Build history of the part. All positions in model axes, mm. A direction names the side the tool comes from. Coordinates: 2 decimals unless noted, no trailing zeros. Order: outer loops, then holes, each group sorted by start corner. A loop starts at its lowest first (then second) coordinate and runs counter-clockwise, first axis right, second up. Notation, with made-up numbers: (29.25, 56.25) - (48.25, 56.25) arc R13 cw to (48.25, 69.25) - close; hole circle Ø8 at (37, -10.5). An arc over 180 degrees is marked (long way). One line per item, written item: value.
from build123d import *

# Parameters (mm, degrees)
SKETCH1_W           = 120
SKETCH1_H           = 120
BOSS_EXTRUDE1_DEPTH = 50
SKETCH3_R           = 35
BOSS_EXTRUDE2_DEPTH = 25
SKETCH4_R           = 25
CUT_EXTRUDE1_DEPTH  = 76
FILLET1_R           = 10
SHELL1_T            = -2
FILLET8_R           = 1.5
FILLET9_R           = 5


with BuildPart() as part:
    # Sketch1 → Boss-Extrude1 (new body)
    with BuildSketch(Plane.XY):
        with Locations((60, 60)):
            Rectangle(SKETCH1_W, SKETCH1_H)
    extrude(amount=BOSS_EXTRUDE1_DEPTH)

    # Sketch3 → Boss-Extrude2 (add)
    with BuildSketch(Plane.XY.offset(50)):
        with Locations((60, 60)):
            Circle(SKETCH3_R)
    extrude(amount=BOSS_EXTRUDE2_DEPTH)

    # Sketch4 → Cut-Extrude1 (cut, through all)
    with BuildSketch(Plane.XY.offset(75)):
        with Locations((60, 60)):
            Circle(SKETCH4_R)
    extrude(amount=-CUT_EXTRUDE1_DEPTH, mode=Mode.SUBTRACT)

    # Fillet1
    fillet1_edges = [part.edges().sort_by_distance(p)[0] for p in [
        (0, 120, 25),
        (120, 120, 25),
        (120, 0, 25),
        (0, 0, 25),
    ]]
    fillet(fillet1_edges, radius=FILLET1_R)

    # Shell1
    shell1_openings = [part.faces().sort_by_distance(p)[0] for p in [
        (85, 60, 0),
    ]]
    offset(amount=SHELL1_T, openings=shell1_openings, kind=Kind.INTERSECTION)

    # Fillet8
    fillet8_edges = [part.edges().sort_by_distance(p)[0] for p in [
        (25, 60, 75),
        (35, 60, 75),
    ]]
    fillet(fillet8_edges, radius=FILLET8_R)

    # Fillet9
    fillet9_edges = [part.edges().sort_by_distance(p)[0] for p in [
        (25, 60, 50),
        (60, 0, 50),
        (0, 60, 50),
        (120, 60, 50),
        (60, 120, 50),
        (117.071067812, 117.071067812, 50),
        (117.071067812, 2.928932188, 50),
        (2.928932188, 117.071067812, 50),
        (2.928932188, 2.928932188, 50),
    ]]
    fillet(fillet9_edges, radius=FILLET9_R)


solid = part.part
1. Band-saw the part on D-D, the plane x = 11.5. Give the cut face in (y, z).
Values found:
outline: (0, 0) - (2, 0) - (2, 48) - (118, 48) - (118, 0) - (120, 0) - (120, 45) arc R5 ccw to (115, 50) - (5, 50) arc R5 ccw to (0, 45) - close
2. Probe line 1 along Y through (x, z) = (60, 43); line 2 along Y through (x, z) = (60, 63.75); line 3 along X through (y, z) = (99, 31). List the from-to ranges inside material, lowest first.
Values found:
line 1: y = 0 to 2, 33 to 35, 85 to 87, 118 to 120
line 2: y = 25 to 27, 33 to 35, 85 to 87, 93 to 95
line 3: x = 0 to 2, 118 to 120
3. Flat gauge pins, fed straight in: P1, Ø2, axis at x = 83.5, z = 60.5, coming from the +Y side; P2, Ø1, axis at x = 20, y = 15, coming from the -Z side; P3, Ø5, axis at x = 99.5, y = 94.5, coming from the +Z side. Where does each tip first touch, or does it go through?
Values found:
P1: stops at y = 86.81
P2: stops at z = 48
P3: stops at z = 50
4. 3-axis set-ups, long thin cutter, end or side, ignore diameter. For faces 4 (the face through (84.94, 49.66, 37.01)), 5 (the face through (35, 97, 50)), 6 (the face through (2, 59, 49)): which of +Z, -Z, +X, -X, +Y, -Y reach the whole face in a straight line?
Values found:
face 4: -Z
face 5: +Z
face 6: +Z, -X, +Y, -Y
5. Two-plate mould, pull along Y, no slides. Class faces 1 (the face through (85, 70, 75)), 2 (the face through (75.227, 30.723, 60.325)), 3 (the face through (61, 2, 49)): pulls with the +Y half, pulls with the -Y half, needs draft (parallel to the pull), parting line crosses it, or undercut.
Values found:
face 1: needs draft
face 2: undercut
face 3: pulls with the -Y half
6. Band-saw the part on A-A, the plane z = 10. Give the cut face in (x, y).
Values found:
outline: (0, 10) arc R10 ccw to (10, 0) - (110, 0) arc R10 ccw to (120, 10) - (120, 110) arc R10 ccw to (110, 120) - (10, 120) arc R10 ccw to (0, 110) - close; circle Ø54 at (60, 60); hole (2, 10) arc R8 ccw to (10, 2) - (110, 2) arc R8 ccw to (118, 10) - (118, 110) arc R8 ccw to (110, 118) - (10, 118) arc R8 ccw to (2, 110) - close; hole circle Ø50 at (60, 60)
